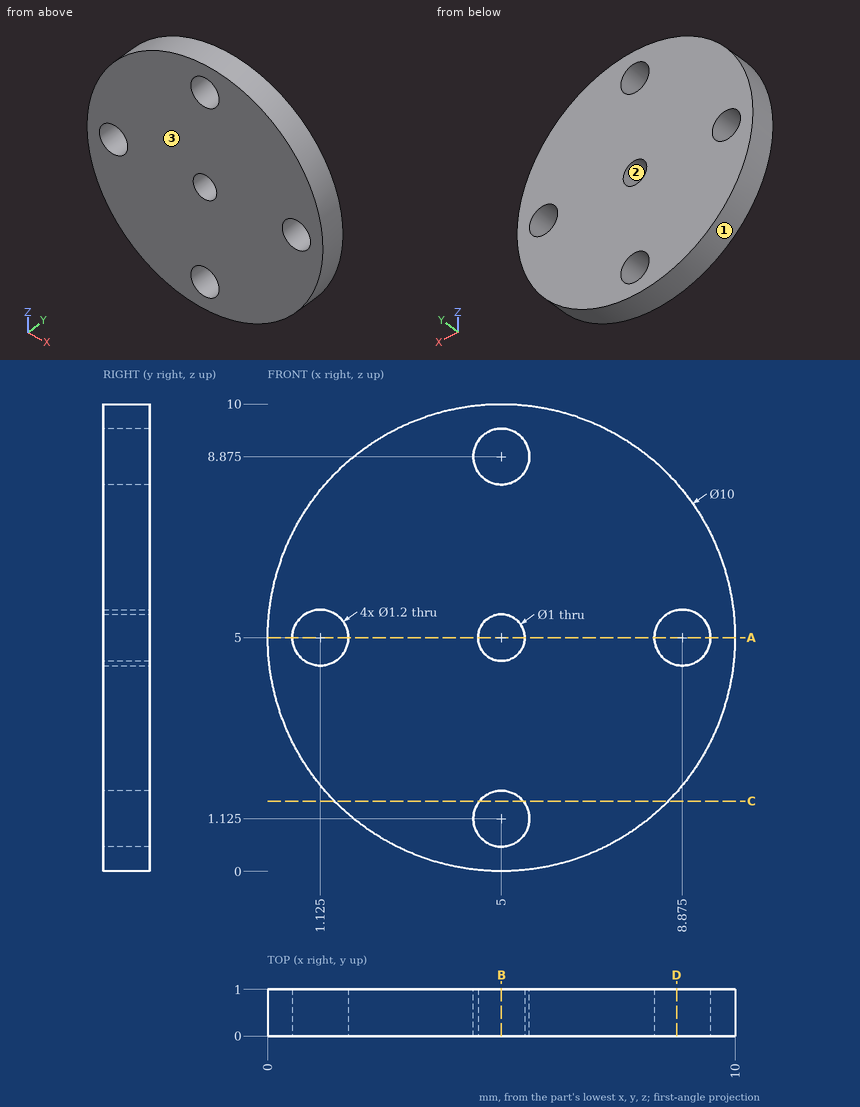
Can you work these out from the drawing? Everything is in mm from the part's minimum corner. Give positions to 0.01 mm unless a question says otherwise; leave off trailing zeros. Write each loop counter-clockwise with the first axis right and the second up, starting at its lowest first coordinate (ties: lowest second). Pieces come first, ordered by that corner, then holes. Notation, with made-up numbers: M 88,47.5 L 94,47.5 A23 cw 94,76.5 Z; hole C 67,58.25 d2. An arc over 180 degrees is marked long. Answer in a Markdown table with one row per item. Add a question column.
Item 1: Please list where these lines run through material, in increasing order: L1, parallel to X at y = 0.75, z = 5 (3 decimals); L2, parallel to X at y = 0.6, z = 4.75; L3, parallel to X at y = 0.5, z = 1.5.
Item 2: For pin 1 Ø0.7 at (x, z) = (1.125, 5) entering from -Y, with a flat end and sliding along its axis, tell me the tip position at first contact or that it passes through.
Item 3: Imagine slicing it at C-C, the plane z = 1.5. Write out the boundary of the cut face in (x, y).
Item 4: Imagine slicing it at B-B, the plane x = 5. Write out the boundary of the cut face in (y, z) (3 decimals), plus the area to 3 significant figures.
Item 5: We'd pull the mould along Z, two halves only. Please class the marked faces 1, 2 and 3: released by +Z, released by -Z, zero draft, split by the parting line, or undercut.
Item 6: Imagine slicing it at A-A, the plane z = 5. Write out the boundary of the cut face in (x, y) (3 decimals).
Item 7: Imagine slicing it at D-D, the plane x = 8.75. Write out the boundary of the cut face in (y, z).
Evaluation:
| question | item | result |
|---|---|---|
| 1 | L1 | x = 0 to 0.525, 1.725 to 4.5, 5.5 to 8.275, 9.475 to 10 |
| 1 | L2 | x = 0.01 to 0.58, 1.67 to 4.57, 5.43 to 8.33, 9.42 to 9.99 |
| 1 | L3 | x = 1.43 to 4.53, 5.47 to 8.57 |
| 2 | pin 1 | passes through |
| 3 | outline | M 1.43,0 L 4.53,0 L 4.53,1 L 1.43,1 Z; M 5.47,0 L 8.57,0 L 8.57,1 L 5.47,1 Z |
| 4 | outline | M 0,0 L 1,0 L 1,0.525 L 0,0.525 Z; M 0,1.725 L 1,1.725 L 1,4.5 L 0,4.5 Z; M 0,5.5 L 1,5.5 L 1,8.275 L 0,8.275 Z; M 0,9.475 L 1,9.475 L 1,10 L 0,10 Z |
| 4 | area | 6.60 mm² |
| 5 | face 1 | split by the parting line |
| 5 | face 2 | undercut |
| 5 | face 3 | zero draft |
| 6 | outline | M 0,0 L 0.525,0 L 0.525,1 L 0,1 Z; M 1.725,0 L 4.5,0 L 4.5,1 L 1.725,1 Z; M 5.5,0 L 8.275,0 L 8.275,1 L 5.5,1 Z; M 9.475,0 L 10,0 L 10,1 L 9.475,1 Z |
| 7 | outline | M 0,1.69 L 1,1.69 L 1,4.41 L 0,4.41 Z; M 0,5.59 L 1,5.59 L 1,8.31 L 0,8.31 Z |
